Could you check a few things on this drawing? It's one solid part, dimensions in mm from its lowest x, y, z. Round coordinates to 2 decimals unless told otherwise and drop trailing zeros. Order: outer loops, then holes, each group sorted by start corner. A loop starts at its lowest first (then second) coordinate and runs counter-clockwise, first axis right, second up. Notation, with made-up numbers: (27, 53) - (57, 53) arc R36 cw to (57, 89) - close; hole circle Ø3 at (-19, 48). An arc over 180 degrees is marked (long way). Use one line per item in the form item = value.
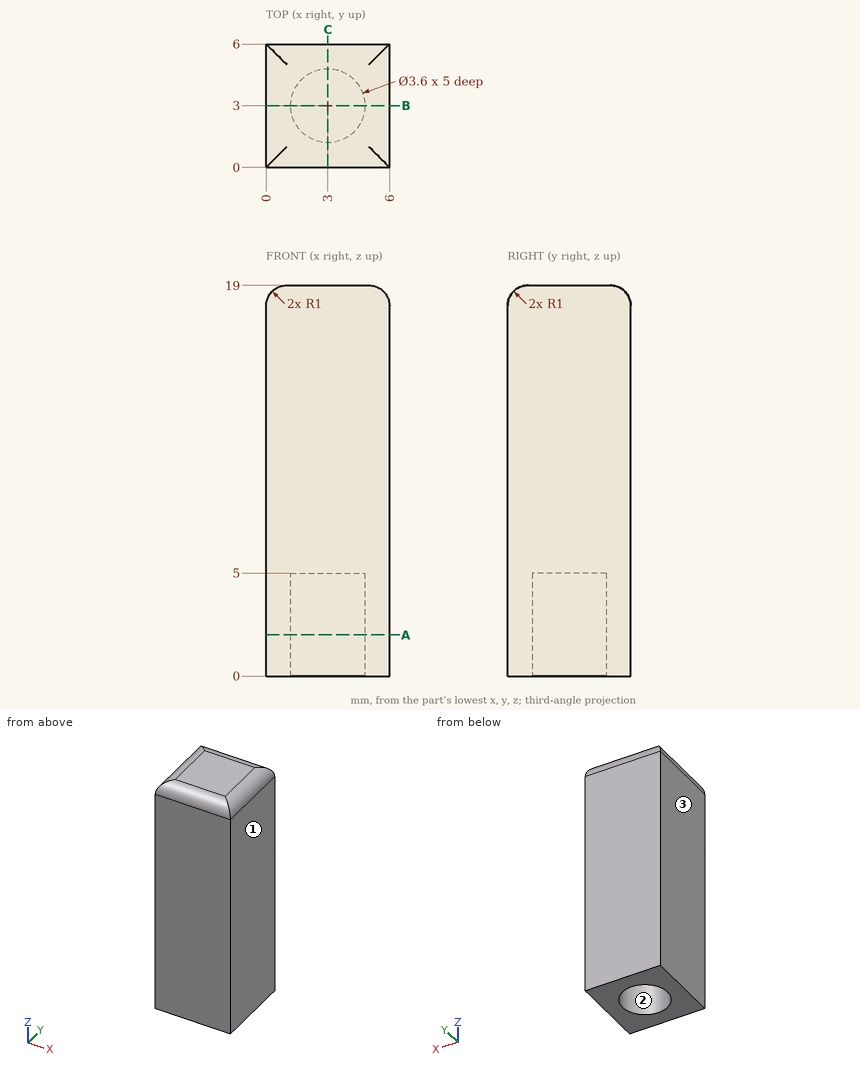
Item 1: If we mould it in two halves opening along X, with no side actions, what happens to the marked faces 1, 2 and 3? For each: released by +X, released by -X, zero draft, split by the parting line, or undercut.
Found:
face_1 = released by +X
face_2 = undercut
face_3 = released by -X
Item 2: Imagine slicing it at B-B on y = 3. Please give me the cut outline in (x, z), plus the area to 3 significant figures.
Found:
outline = (0, 0) - (1.2, 0) - (1.2, 5) - (4.8, 5) - (4.8, 0) - (6, 0) - (6, 18) arc R1 ccw to (5, 19) - (1, 19) arc R1 ccw to (0, 18) - close
area = 95.6 mm2
Item 3: I need wall thicknesses on L1, parallel to Y at x = 3, z = 2.25; L2, parallel to Z at x = 2.4, y = 3.95; L3, parallel to Z at x = 5.05, y = 2. Which ranges of each line are inside material? Lowest first, please.
Found:
L1 = 0 to 1.2, 4.8 to 6
L2 = 5 to 19
L3 = 0 to 19
Item 4: Imagine slicing it at A-A on z = 2. Please give me the cut outline in (x, y).
Found:
outline = (0, 0) - (6, 0) - (6, 6) - (0, 6) - close; hole circle Ø3.6 at (3, 3)
Item 5: Will this pin go through, and if not, where does the flat tip stop? P1, Ø1.1, axis at x = 3, y = 3, coming from the -Z side.
Found:
P1 = 5
